Design review of the part built by this model. Coordinates are the model's own, in mm. A direction names the side the tool comes from. Coordinates: 2 decimals unless noted, no trailing zeros. Write each loop counter-clockwise with the first axis right and the second up, starting at its lowest first coordinate (ties: lowest second). Pieces come first, ordered by that corner, then holes.
Q1. Take a section at A-A, the plane z = 1917.5. Write out the cut boundary in (x, y).
Q2. For pin 1 Ø25 at (y, z) = (17.5, 754.5) entering from +X; pin 2 Ø1.6 at (x, z) = (19.5, 734.5) entering from -Y; pin 3 Ø3 at (x, z) = (-0.5, 1041) entering from +Y, all flat-tipped, find the tip position at first contact; note any pin that passes through.
Q3. For L1, parallel to Z at x = -1.5, y = 38; L2, parallel to X at y = 27, z = 1040 (3 decimals); L3, parallel to Z at x = -2, y = 34, list the stretches that pass through material, from the lowest coordinate up.
Q4. For faces 1 (the flat face through (-17.5, -1, 1025)), 2 (the flat face through (17.5, -23, 1025)), list the 3-axis set-ups (+Z, -Z, +X, -X, +Y, -Y) from which the entire face can be reached by the end or side of a thin tool; tool diameter is ignored.
from build123d import *

# Parameters (mm, degrees)
SALIENTE_EXTRUIR1_DEPTH = 2080
CROQUIS2_R              = 3.175
CORTAR_EXTRUIR1_DEPTH   = 30


with BuildPart() as part:
    # Croquis1 → Saliente-Extruir1 (new body)
    with BuildSketch(Plane.XY):
        Polygon((17.5, 50), (20.5, 50), (20.5, 45.5), (19, 45.5), (19, 48.5), (17.5, 48.5), (17.5, -1.5), (19, -1.5), (19, 1.5), (20.5, 1.5), (20.5, -3), (17.5, -3), (17.5, -44), (20.5, -44), (20.5, -48.5), (19, -48.5), (19, -45.5), (17.5, -45.5), (17.5, -50), (-17.5, -50), (-17.5, 50), align=None)
    extrude(amount=SALIENTE_EXTRUIR1_DEPTH)

    # Croquis2 → Cortar-Extruir1 (cut)
    with BuildSketch(Plane(origin=(0, 50, 0), x_dir=(1, 0, 0), z_dir=(0, 1, 0))):
        with Locations(Location((0, -20, 0), (0, 0, 270))):
            Circle(CROQUIS2_R)
        with Locations(Location((0, -1040, 0), (0, 0, 270))):
            Circle(CROQUIS2_R)
        with Locations(Location((0, -2060, 0), (0, 0, 270))):
            Circle(CROQUIS2_R)
    extrude(amount=-CORTAR_EXTRUIR1_DEPTH, mode=Mode.SUBTRACT)


solid = part.part
Responses:
1. outline: (-17.5, -50) - (17.5, -50) - (17.5, -45.5) - (19, -45.5) - (19, -48.5) - (20.5, -48.5) - (20.5, -44) - (17.5, -44) - (17.5, -3) - (20.5, -3) - (20.5, 1.5) - (19, 1.5) - (19, -1.5) - (17.5, -1.5) - (17.5, 48.5) - (19, 48.5) - (19, 45.5) - (20.5, 45.5) - (20.5, 50) - (-17.5, 50) - close
2. pin 1: stops at x = 17.5
2. pin 2: stops at y = -48.5
2. pin 3: stops at y = 20
3. L1: z = 0 to 17.2, 22.8 to 1037.2, 1042.8 to 2057.2, 2062.8 to 2080
3. L2: x = -17.5 to -3.175, 3.175 to 17.5
3. L3: z = 0 to 17.53, 22.47 to 1037.53, 1042.47 to 2057.53, 2062.47 to 2080
4. face 1: +Z, -Z, -X, +Y, -Y
4. face 2: +Z, -Z, +X
